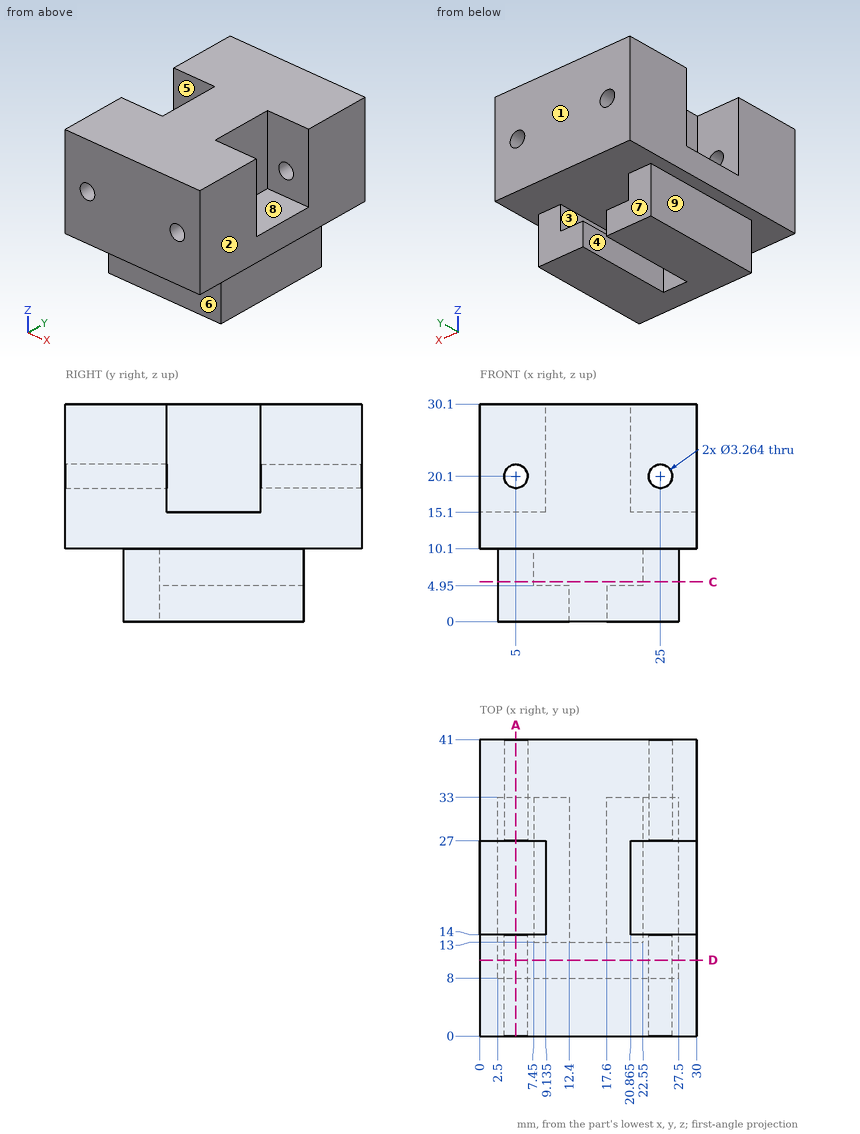
Answer from the drawing. Dimensions are ordinates in mm from the lowest x, y and z of the part. A direction names the side the tool comes from. Coordinates: 2 decimals unless noted, no trailing zeros. Order: outer loops, then holes, each group sorted by start corner. A loop starts at its lowest first (then second) coordinate and runs counter-clockwise, first axis right, second up. Notation, with made-up numbers: M -24.75,11 L -19.75,11 A23 ccw -19.75,45 Z; hole C 46,82.25 d8. An arc over 180 degrees is marked long. Put each result on its own line as item: value. Start each with the question number.
Item 1: For the marked faces 5, 6, 7, 8 and 9, determine the directions among +Z, -Z, +X, -X, +Y, -Y from which every point of the face is accessible in a straight line to the end or side of a thin tool.
Item 2: Section C-C, the plane z = 5.5 is taken. Determine the outline of the cut face in (x, y), plus the area to 3 significant figures.
Item 3: Consider probe 1 along Y at (x, z) = (23, 29); probe 2 along X at (y, z) = (30, 20); probe 3 along X at (y, z) = (27.5, 8.5). Determine where each line is inside the solid, lowest interval first. Write a range as [from, to].
Item 4: Section A-A, the plane x = 5 is taken. Determine the outline of the cut face in (y, z).
Item 5: The mould has two halves that part along X. Classify the marked faces 1, 2, 3 and 4: +X half, -X half, draft (parallel to the pull), parting line (faces both ways), or undercut.
Item 6: Given pin 1 Ø1.5 at (y, z) = (20.5, 1.5) entering from +X; pin 2 Ø1 at (x, z) = (14.5, 7) entering from -Y; pin 3 Ø3 at (y, z) = (25, 3) entering from -X, each flat-ended and moving along its own axis, determine where each tip first touches the part or whether it passes through.
Item 7: Section D-D, the plane y = 10.5 is taken. Determine the outline of the cut face in (x, z).
Computed:
1. face 5: +Z, -X
1. face 6: -Z, +X, -X, -Y
1. face 7: -Z, +X, -X, +Y
1. face 8: +Z, +X
1. face 9: -Z, -X, +Y, -Y
2. outline: M 2.5,8 L 27.5,8 L 27.5,33 L 22.55,33 L 22.55,13 L 7.45,13 L 7.45,33 L 2.5,33 Z
2. area: 323 mm2
3. probe 1: y = [0, 14], [27, 41]
3. probe 2: x = [0, 3.37], [6.63, 23.37], [26.63, 30]
3. probe 3: x = [2.5, 7.45], [22.55, 27.5]
4. outline: M 0,10.1 L 8,10.1 L 8,0 L 33,0 L 33,10.1 L 41,10.1 L 41,18.47 L 27,18.47 L 27,15.1 L 14,15.1 L 14,18.47 L 0,18.47 Z; M 0,21.73 L 14,21.73 L 14,30.1 L 0,30.1 Z; M 27,21.73 L 41,21.73 L 41,30.1 L 27,30.1 Z
5. face 1: draft
5. face 2: +X half
5. face 3: undercut
5. face 4: undercut
6. pin 1: stops at x = 27.5
6. pin 2: stops at y = 8
6. pin 3: stops at x = 2.5
7. outline: M 0,10.1 L 2.5,10.1 L 2.5,0 L 27.5,0 L 27.5,10.1 L 30,10.1 L 30,30.1 L 0,30.1 Z; hole C 5,20.1 d3.26; hole C 25,20.1 d3.26
